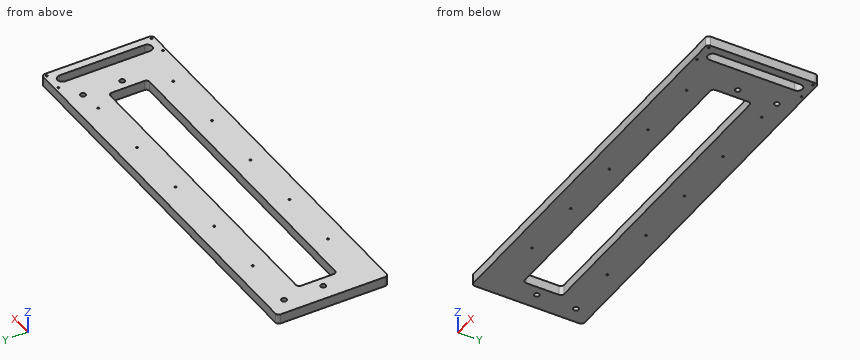
from build123d import *

# Parameters (mm, degrees)
SKETCH2_W                   = 723.9
SKETCH2_H                   = 215.9
BOSS_EXTRUDE1_DEPTH         = 19.05
CUT_EXTRUDE3_DEPTH          = 409.675659906
F_27_0_144_DIAMETER_HOLE1_D = 3.6576
F_3_8_CLEARANCE_HOLE1_D     = 10.0838
SKETCH22_W                  = 19.05
SKETCH22_H                  = 215.9
BOSS_EXTRUDE2_DEPTH         = 50.8
FILLET1_R                   = 6.35
F_6_CLEARANCE_HOLE1_D       = 3.6576
CUT_EXTRUDE4_DEPTH          = 76.2


with BuildPart() as part:
    # Sketch2 → Boss-Extrude1 (new body)
    with BuildSketch(Plane.XY):
        with Locations((-31.75, 0)):
            Rectangle(SKETCH2_W, SKETCH2_H)
    extrude(amount=BOSS_EXTRUDE1_DEPTH)

    # Sketch13 → Cut-Extrude3 (cut, through all)
    with BuildSketch(Plane.XY.offset(19.05)):
        with BuildLine():
            Line((-336.55, -38.1), (273.05, -38.1))
            ThreePointArc((273.05, -38.1), (277.540128061, -36.240128061), (279.4, -31.75))
            Line((279.4, -31.75), (279.4, 31.75))
            ThreePointArc((279.4, 31.75), (277.540128061, 36.240128061), (273.05, 38.1))
            Line((273.05, 38.1), (-336.55, 38.1))
            ThreePointArc((-336.55, 38.1), (-341.040128061, 36.240128061), (-342.9, 31.75))
            Line((-342.9, 31.75), (-342.9, -31.75))
            ThreePointArc((-342.9, -31.75), (-341.040128061, -36.240128061), (-336.55, -38.1))
        make_face()
    extrude(amount=-CUT_EXTRUDE3_DEPTH, mode=Mode.SUBTRACT)

    # #27 (0.144) Diameter Hole1 (through all)
    with Locations(Plane(origin=(0, 0, 0), x_dir=(-1, 0, 0), z_dir=(0, 0, -1))):
        with Locations((0, 0), (-254, 73.025), (-127, 73.025), (0, 73.025), (127, 73.025), (254, 73.025), (-127, -73.025), (0, -73.025), (127, -73.025), (254, -73.025), (-254, -73.025)):
            Hole(F_27_0_144_DIAMETER_HOLE1_D / 2)

    # 3/8 Clearance Hole1 (through all)
    with Locations(Plane(origin=(0, 0, 0), x_dir=(-1, 0, 0), z_dir=(0, 0, -1))):
        with Locations((-298.45, 76.2), (361.95, 76.2), (361.95, 0), (-298.45, 0)):
            Hole(F_3_8_CLEARANCE_HOLE1_D / 2)

    # Sketch22 → Boss-Extrude2 (add)
    with BuildSketch(Plane(origin=(330.2, 0, 0), x_dir=(0, 0, -1), z_dir=(1, 0, 0))):
        with Locations((-9.525, 0)):
            Rectangle(SKETCH22_W, SKETCH22_H)
    extrude(amount=BOSS_EXTRUDE2_DEPTH)

    # Fillet1
    fillet1_edges = [part.edges().sort_by_distance(p)[0] for p in [
        (381, -107.95, 9.525),
        (381, 107.95, 9.525),
        (-393.7, 107.95, 9.525),
        (-393.7, -107.95, 9.525),
    ]]
    fillet(fillet1_edges, radius=FILLET1_R)

    # #6 Clearance Hole1 (through all)
    with Locations(Plane.XY.offset(19.05)):
        with Locations((336.55, -101.6), (355.6, 0), (336.55, 101.6), (374.65, -101.6), (374.65, 101.6)):
            Hole(F_6_CLEARANCE_HOLE1_D / 2)

    # Sketch25 → Cut-Extrude4 (cut)
    with BuildSketch(Plane.XY.offset(19.05)):
        with BuildLine():
            Line((346.075, -82.55), (346.075, 82.55))
            ThreePointArc((346.075, 82.55), (355.6, 92.075), (365.125, 82.55))
            Line((365.125, 82.55), (365.125, -82.55))
            ThreePointArc((365.125, -82.55), (355.6, -92.075), (346.075, -82.55))
        make_face()
    extrude(amount=-CUT_EXTRUDE4_DEPTH, mode=Mode.SUBTRACT)


solid = part.part
Can you work these out from the model? Positions are in its coordinate system, mm. Round coordinates to 2 decimals unless told otherwise and drop trailing zeros. Write each loop counter-clockwise with the first axis right and the second up, starting at its lowest first coordinate (ties: lowest second). Pieces come first, ordered by that corner, then holes. Notation, with made-up numbers: (-18.5, 19.25) -> (23.5, 19.25) arc R11 cw to (23.5, 24.25) -> close; hole circle Ø4 at (64.5, -38). An arc over 180 degrees is marked (long way). One line per question, with ' | ' between items. Start each with the question number.
1) Suppose I cut it at C-C on z = 10. Count the separate pieces of the cut face and the enclosed holes in it, then the cut area to 3 significant figures.
2) Suppose I cut it at A-A on x = 355.6. Write out the boundary of the cut face in (y, z) (3 decimals), then the cut area to 3 significant figures.
3) I need wall thicknesses on line 1 (X direction, y = 22, z = 14.75) (3 decimals); line 2 (Y direction, x = 127, z = 7.75); line 3 (Y direction, x = 336.55, z = 9.25). Which ranges of each line are inside material? Lowest first, please. Write a range as [from, to].
4) Suppose I cut it at B-B on x = -309. Write out the boundary of the cut face in (y, z), then the cut area to 3 significant figures.
Return value:
1) separate pieces: 1 | enclosed holes: 20 | area: 116,000 mm2
2) outline: (-107.95, 0) -> (-92.075, 0) -> (-92.075, 19.05) -> (-107.95, 19.05) -> close; (92.075, 0) -> (107.95, 0) -> (107.95, 19.05) -> (92.075, 19.05) -> close | area: 605 mm2
3) line 1: x = [-393.7, -342.9], [279.4, 346.075], [365.125, 381] | line 2: y = [-107.95, -74.85], [-71.2, -38.1], [38.1, 71.2], [74.85, 107.95] | line 3: y = [-107.95, -103.43], [-99.77, 99.77], [103.43, 107.95]
4) outline: (-107.95, 0) -> (-38.1, 0) -> (-38.1, 19.05) -> (-107.95, 19.05) -> close; (38.1, 0) -> (107.95, 0) -> (107.95, 19.05) -> (38.1, 19.05) -> close | area: 2,660 mm2
